```python
from build123d import *

# Parameters (mm, degrees)
CROQUIS1_R              = 2
SALIENTE_EXTRUIR1_DEPTH = 3


with BuildPart() as part:
    # Croquis1 → Saliente-Extruir1 (new body)
    with BuildSketch(Plane.XY):
        with BuildLine():
            Line((-4.5, 85), (-4.5, 0))
            ThreePointArc((-4.5, 0), (0, -4.5), (4.5, 0))
            Line((4.5, 0), (4.5, 85))
            ThreePointArc((4.5, 85), (0, 89.5), (-4.5, 85))
        make_face()
        with Locations((0, 85)):
            Circle(CROQUIS1_R, mode=Mode.SUBTRACT)
        Circle(CROQUIS1_R, mode=Mode.SUBTRACT)
        with BuildLine():
            Line((-2, 75), (-2, 10))
            ThreePointArc((-2, 10), (0, 8), (2, 10))
            Line((2, 10), (2, 75))
            ThreePointArc((2, 75), (0, 77), (-2, 75))
        make_face(mode=Mode.SUBTRACT)
    extrude(amount=SALIENTE_EXTRUIR1_DEPTH)


solid = part.part
```
Geometry: final body of the model. Coordinates: model frame, mm. A direction names the side the tool comes from. Round coordinates to 2 decimals unless told otherwise and drop trailing zeros. Order: outer loops, then holes, each group sorted by start corner. A loop starts at its lowest first (then second) coordinate and runs counter-clockwise, first axis right, second up. Notation, with made-up numbers: M 76.5,58 L 135.5,58 A24 ccw 135.5,81 Z; hole C 49,5 d6. An arc over 180 degrees is marked long. Use one line per item in the form item = value. Start each with the question number.
Q1. Access query for faces 1 (the face through (-2, 43, 1)), 2 (the face through (4.5, 42, 1)). Directions: +Z, -Z, +X, -X, +Y, -Y. A direction counts if a zero-diameter tool reaches every point of the face in a straight line with its end or side. Return the directions, or none.
Q2. Pin query (flat end, axial travel): pin 1 Ø1 at (x, y) = (-0.5, 78) entering from -Z. Return the tip coordinate at first contact, or that it passes through.
Q3. Cut plane C-C (z = 1.45). Return loops of the section in (x, y).
Q4. Cut plane A-A (x = 0). Return loops of the section in (y, z).
Q5. Cut plane B-B (y = 58.5). Return loops of the section in (x, z), and give its area (3 significant figures).
Q6. Material intervals for line 1 (Y direction, x = 0, z = 2); line 2 (X direction, y = 40, z = 1.65); line 3 (Y direction, x = -0.5, z = 1.8), sorted ascending. Write a range as [from, to].
Q7. Mould query, pull axis Y, two halves, no side actions, for faces 3 (the face through (0.1, 89.5, 1.5)), 4 (the face through (-4.5, 43, 1)), 5 (the face through (2, 42, 1)), 6 (the face through (-0.1, -4.5, 1.5)). Classes: +Y half, -Y half, draft (parallel to the pull), parting line (faces both ways), or undercut.
Geometry results:
q1.face_1 = +Z, -Z
q1.face_2 = +Z, -Z, +X, +Y, -Y
q2.pin_1 = 0
q3.outline = M -4.5,0 A4.5 ccw 4.5,0 L 4.5,85 A4.5 ccw -4.5,85 Z; hole C 0,0 d4; hole M -2,10 A2 ccw 2,10 L 2,75 A2 ccw -2,75 Z; hole C 0,85 d4
q4.outline = M -4.5,0 L -2,0 L -2,3 L -4.5,3 Z; M 2,0 L 8,0 L 8,3 L 2,3 Z; M 77,0 L 83,0 L 83,3 L 77,3 Z; M 87,0 L 89.5,0 L 89.5,3 L 87,3 Z
q5.outline = M -4.5,0 L -2,0 L -2,3 L -4.5,3 Z; M 2,0 L 4.5,0 L 4.5,3 L 2,3 Z
q5.area = 15.0 mm^2
q6.line_1 = [-4.5, -2], [2, 8], [77, 83], [87, 89.5]
q6.line_2 = [-4.5, -2], [2, 4.5]
q6.line_3 = [-4.47, -1.94], [1.94, 8.06], [76.94, 83.06], [86.94, 89.47]
q7.face_3 = +Y half
q7.face_4 = draft
q7.face_5 = undercut
q7.face_6 = -Y half
